CAD build for the part. Positions are in the model's coordinates, mm. Face numbers are marked on the shaded views. A direction names the side the tool comes from. Coordinates: 2 decimals unless noted, no trailing zeros. Order: outer loops, then holes, each group sorted by start corner. A loop starts at its lowest first (then second) coordinate and runs counter-clockwise, first axis right, second up.
Autodesk Inventor part; units mm, degrees
ref_plane "YZ Plane" through (0, 0, 0) normal (1, 0, 0) x (0, 1, 0)
ref_plane "XZ Plane" through (0, 0, 0) normal (0, 1, 0) x (-1, 0, 0)
ref_plane "XY Plane" through (0, 0, 0) normal (0, 0, 1) x (1, 0, 0)
sketch "Sketch1" plane through (0, 0, 0) normal (0, 0, 1) x (1, 0, 0)
  circle A0 centre (9.329895, 6.999479) radius 4
  line L0 (9.329895, 6.999479) -> (-2.391324, -17.323617)
  circle A1 centre (51.212876, -35.96348) radius 4
  line L1 (9.329895, 6.999479) -> (-2.391324, -17.323617) construction
  line L2 (7.753398, 7.759188) -> (-3.967821, -16.563909)
  line L3 (-0.814827, -18.083326) -> (10.906392, 6.239771)
  arc A2 (10.906392, 6.239771) -> (7.753398, 7.759188) centre (9.329895, 6.999479) ccw
  arc A3 (-3.967821, -16.563909) -> (-0.814827, -18.083326) centre (-2.391324, -17.323617) ccw
  arc A4 (-2.542999, -15.580203) -> (-2.239649, -19.067032) centre (-2.391324, -17.323617) ccw
  arc A5 (49.95979, -37.185067) -> (52.465962, -34.741893) centre (51.212876, -35.96348) ccw
  arc A6 (49.95979, -37.185067) -> (-2.239649, -19.067032) centre (2.770217, -88.887525) ccw
  arc A7 (52.465962, -34.741893) -> (-2.542999, -15.580203) centre (4.022714, -85.271604) ccw
  point P0 (0, 0)
  point P1 (3.469285, -5.162069)
  point P2 (47.351434, -34.919803)
  point P3 (49.725474, -32.250309)
  point P4 (0.497325, -15.360435)
  point P5 (9.34492, 2.999507)
  point P6 (6.191926, 4.518925)
  point P7 (-2.239649, -19.067032)
  dimension "d0" = 8
  dimension "d1" = 27
  dimension "d3" = 8
  dimension "d4" = 3.5
  dimension "d6" = 3.5
  dimension "d7" = 70
  dimension "d8" = 70
extrude "Extrusion1" add sketch "Sketch1" along normal blind 7
sketch "Sketch2" plane through (0, 0, 7) normal (0, 0, 1) x (1, 0, 0)
  line L0 (0.497325, -15.360435) -> (9.34492, 2.999507)
  arc A0 (9.34492, 2.999507) -> (6.191926, 4.518925) centre (9.329895, 6.999479) ccw
  line L1 (6.191926, 4.518925) -> (-3.967821, -16.563909)
  arc A1 (-3.967821, -16.563909) -> (-2.239649, -19.067032) centre (-2.391324, -17.323617) ccw
  arc A2 (47.351434, -34.919803) -> (-2.239649, -19.067032) centre (2.770217, -88.887525) ccw
  arc A3 (47.351434, -34.919803) -> (49.725474, -32.250309) centre (51.212876, -35.96348) ccw
  arc A4 (49.725474, -32.250309) -> (0.497325, -15.360435) centre (4.022714, -85.271604) ccw
  point P0 (0, 0)
hole "Hole1" at (51.212876, -35.96348, 7) at (9.329895, 6.999479, 7) direction (0, 0, -1) diameter 3 depth 8
sketch "Sketch3" plane through (0, 0, 0) normal (0, 0, -1) x (-1, 0, 0)
  circle A0 centre (-51.212876, -35.96348) radius 1.5
  circle A1 centre (-9.329895, 6.999479) radius 1.5
  line L0 (-0.497325, -15.360435) -> (-9.34492, 2.999507)
  arc A2 (-0.497325, -15.360435) -> (-49.725474, -32.250309) centre (-4.022714, -85.271604) ccw
  arc A3 (-49.725474, -32.250309) -> (-47.351434, -34.919803) centre (-51.212876, -35.96348) ccw
  arc A4 (2.239649, -19.067032) -> (-47.351434, -34.919803) centre (-2.770217, -88.887525) ccw
  arc A5 (2.239649, -19.067032) -> (3.967821, -16.563909) centre (2.391324, -17.323617) ccw
  line L1 (-6.191926, 4.518925) -> (3.967821, -16.563909)
  arc A6 (-6.191926, 4.518925) -> (-9.34492, 2.999507) centre (-9.329895, 6.999479) ccw
  circle A7 centre (-9.329895, 6.999479) radius 4
  circle A8 centre (-51.212876, -35.96348) radius 4
  point P0 (0, 0)
  point P1 (-49.725474, -32.250309)
  dimension "d18" = 8
  dimension "d19" = 8
extrude "Extrusion2" cut sketch "Sketch3" against normal blind 2 contours L0 A7 L1 A5 A4 A8 A2
fillet "Fillet1" radius 2 6 edges at (47.3514, -34.9198, 4.5) (48.2239, -33.3053, 2) (49.7255, -32.2503, 4.5) (9.3449, 2.9995, 4.5) (7.5934, 3.3961, 2) (6.1919, 4.5189, 4.5)
fillet "Fillet2" radius 1 1 edges at (0.4973, -15.3604, 4.5)
properties part number "leg_link_3"
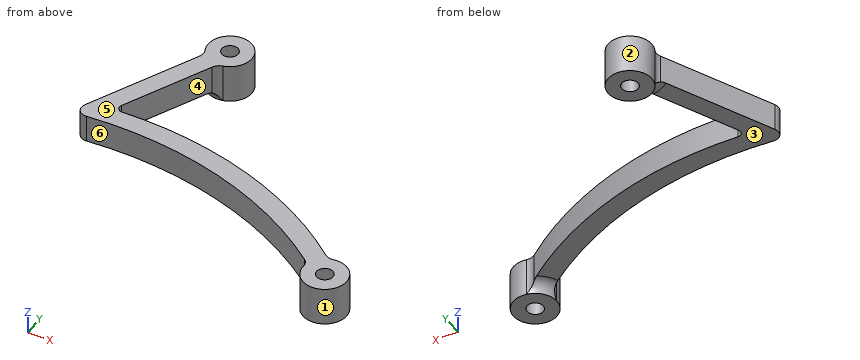
1) Which spindle directions (+Z, -Z, +X, -X, +Y, -Y) get a long thin tool onto all of the face, cutting with end or side? Do the marked faces 4, 5 and 6. Say none if no direction does.
2) Slice it at A-A (z = 1). List the corners of the cut face in (x, y), plus the area to 3 significant figures.
3) Pin check, flat tips, straight feed: P1, Ø3, axis at y = 0.5, z = 3, coming from the -X side; P2, Ø4, axis at y = -28, z = 2, coming from the -X side; P3, Ø2.5, axis at x = 51.21, y = -35.96, coming from the +Z side; P4, Ø4, axis at y = -31.5, z = 6, coming from the +X side. Stop position of each tip, or through.
4) Two-plate mould, pull along Y, no slides. Class the marked faces 1, 2 and 3: released by +Y, released by -Y, zero draft, split by the parting line, or undercut.
5) Slice it at B-B (y = 7). List the corners of the cut face in (x, z), plus the area to 3 significant figures.
6) Slice it at C-C (x = 12). List the corners of the cut face in (y, z).
7) Slice it at D-D (z = 5.25). List the corners of the cut face in (x, y).
8) Drill centre lines: probe 1 along X at (y, z) = (-35, 5.75); probe 2 along Z at (x, y) = (5, -3); probe 3 along Y at (x, z) = (50, 0.5). Where is each one in solid material? Low to high.
Worked out:
1. face 4: +Z, -Z, +X
1. face 5: +Z, +X, -X, +Y, -Y
1. face 6: +Z, -Z, -Y
2. outline: (5.72, 5.27) arc R2 cw to (5.92, 4.44) arc R4.27 ccw to (9.45, 2.73) arc R2 cw to (10.23, 3.1) arc R4 ccw (long way) to start; (47.06, -34.98) arc R2 cw to (47.22, -35.83) arc R4 ccw (long way) to (50.55, -32.02) arc R2 cw to (49.69, -31.98) arc R4.27 ccw to start; hole circle Ø3 at (9.33, 7); hole circle Ø3 at (51.21, -35.96)
2. area: 88.8 mm2
3. P1: stops at x = 3.53
3. P2: stops at x = 33.51
3. P3: passes through
3. P4: stops at x = 54.36
4. face 1: split by the parting line
4. face 2: undercut
4. face 3: zero draft
5. outline: (5.33, 0) - (7.83, 0) - (7.83, 7) - (5.33, 7) - close; (10.83, 0) - (13.33, 0) - (13.33, 7) - (10.83, 7) - close
5. area: 35.0 mm2
6. outline: (-19.5, 2) - (-15.73, 2) - (-15.73, 7) - (-19.5, 7) - close; (4.02, 0) - (9.98, 0) - (9.98, 7) - (4.02, 7) - close
7. outline: (-3.97, -16.56) arc R1.75 ccw to (-2.24, -19.07) arc R70 cw to (46.46, -34.2) arc R2 cw to (47.22, -35.83) arc R4 ccw (long way) to (50.55, -32.02) arc R2 cw to (48.94, -31.58) arc R70 ccw to (2.15, -15.3) arc R1 cw to (1.22, -13.86) - (8.87, 2.02) arc R2 cw to (10.23, 3.1) arc R4 ccw (long way) to (5.72, 5.27) arc R2 cw to (5.72, 3.54) - close; hole circle Ø3 at (9.33, 7); hole circle Ø3 at (51.21, -35.96)
8. probe 1: x = 47.07 to 50.06, 52.36 to 55.1
8. probe 2: z = 2 to 7
8. probe 3: y = -39.78 to -36.85, -35.08 to -32.09
